```python
from build123d import *

# Parameters (mm, degrees)
SKETCH_1_W          = 60
SKETCH_1_H          = 10.5
SKETCH_1_R          = 1.55
EXTRUDE_1_DEPTH     = 77
SKETCH_2_W          = 25
SKETCH_2_H          = 77
EXTRUDE_2_DEPTH     = 8.5
FILLET_2_R          = 4
SKETCH_3_R          = 1.55
CUT_EXTRUDE_1_DEPTH = 8
SKETCH_4_R          = 2.05
CUT_EXTRUDE_2_DEPTH = 5
CUT_EXTRUDE_START   = -5
SKETCH_5_R          = 2.05
CUT_EXTRUDE_3_DEPTH = 5
FILLET_3_R          = 1
SKETCH_6_R          = 2.05
CUT_EXTRUDE_4_DEPTH = 5


with BuildPart() as part:
    # 草图1 → 凸台-拉伸1 (new body)
    with BuildSketch(Plane.XY):
        with Locations((30, 5.25)):
            Rectangle(SKETCH_1_W, SKETCH_1_H)
        with Locations((15, 5.5)):
            Circle(SKETCH_1_R, mode=Mode.SUBTRACT)
        with Locations((45, 5.5)):
            Circle(SKETCH_1_R, mode=Mode.SUBTRACT)
    extrude(amount=EXTRUDE_1_DEPTH)

    # 草图2 → 凸台-拉伸2 (add)
    with BuildSketch(Plane.XZ):
        with Locations((47.5, 38.5)):
            Rectangle(SKETCH_2_W, SKETCH_2_H)
    extrude(amount=EXTRUDE_2_DEPTH)

    # 圆角2
    fillet_2_edges = [part.edges().sort_by_distance(p)[0] for p in [
        (35, 0, 38.5),
        (60, -8.5, 38.5),
        (35, -8.5, 38.5),
        (0, 10.5, 38.5),
        (60, 10.5, 38.5),
        (0, 0, 38.5),
    ]]
    fillet(fillet_2_edges, radius=FILLET_2_R)

    # 草图3 → 切除-拉伸1 (cut)
    with BuildSketch(Plane.XZ):
        with Locations((11.15, 63.5)):
            Circle(SKETCH_3_R)
        with Locations((11.15, 13.5)):
            Circle(SKETCH_3_R)
        with Locations((25.15, 63.5)):
            Circle(SKETCH_3_R)
        with Locations((25.15, 13.5)):
            Circle(SKETCH_3_R)
    extrude(amount=-CUT_EXTRUDE_1_DEPTH, mode=Mode.SUBTRACT)

    # 草图4 → 切除-拉伸2 (cut)
    with BuildSketch(Plane(origin=(0, 0, 0), x_dir=(-1, 0, 0), z_dir=(0, 0, -1))):
        with Locations((-45, 5.5)):
            Circle(SKETCH_4_R)
        with Locations((-15, 5.5)):
            Circle(SKETCH_4_R)
    extrude(amount=-CUT_EXTRUDE_2_DEPTH, mode=Mode.SUBTRACT)

    # 草图5 → 切除-拉伸3 (cut)
    with BuildSketch(Plane.XY.offset(77).offset(CUT_EXTRUDE_START)):
        with Locations(Location((15, 5.5, 0), (0, 0, 180))):
            Circle(SKETCH_5_R)
        with Locations(Location((45, 5.5, 0), (0, 0, 180))):
            Circle(SKETCH_5_R)
    extrude(amount=CUT_EXTRUDE_3_DEPTH, mode=Mode.SUBTRACT)

    # 圆角3
    fillet_3_edges = [part.edges().sort_by_distance(p)[0] for p in [
        (47.5, -8.5, 77),
        (47.5, -8.5, 0),
        (0, 5.25, 0),
        (30, 10.5, 0),
        (60, 1, 0),
        (35, -4.25, 0),
        (17.5, 0, 0),
        (1.171572875, 9.328427125, 0),
        (1.171572875, 1.171572875, 0),
        (58.828427125, 9.328427125, 0),
        (58.828427125, -7.328427125, 0),
        (36.171572875, -7.328427125, 0),
        (35, -4.25, 77),
        (0, 5.25, 77),
        (17.5, 0, 77),
        (60, 1, 77),
        (30, 10.5, 77),
        (1.171572875, 9.328427125, 77),
        (1.171572875, 1.171572875, 77),
        (58.828427125, 9.328427125, 77),
        (58.828427125, -7.328427125, 77),
        (36.171572875, -7.328427125, 77),
        (33.828427125, -1.171572875, 0),
        (33.828427125, -1.171572875, 77),
    ]]
    fillet(fillet_3_edges, radius=FILLET_3_R)

    # 草图6 → 切除-拉伸4 (cut)
    with BuildSketch(Plane.XZ):
        with Locations((11.15, 63.5)):
            Circle(SKETCH_6_R)
        with Locations((25.15, 63.5)):
            Circle(SKETCH_6_R)
        with Locations((25.15, 13.5)):
            Circle(SKETCH_6_R)
        with Locations((11.15, 13.5)):
            Circle(SKETCH_6_R)
    extrude(amount=-CUT_EXTRUDE_4_DEPTH, mode=Mode.SUBTRACT)


solid = part.part
```
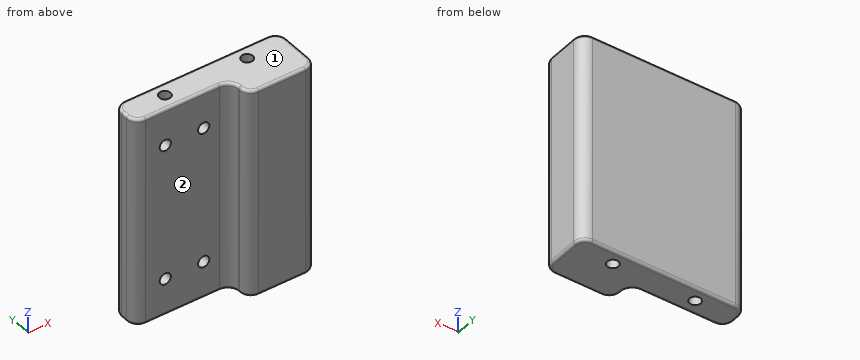
For this review, take the finished solid that the model builds, in its own axes (mm). Face numbers are marked on the shaded views. A direction names the side the tool comes from. Coordinates: 2 decimals unless noted, no trailing zeros. Loops run counter-clockwise (first coordinate to the right, second up) from the corner with the lowest first, then second, coordinate; pieces in that order, holes last. Notation, with made-up numbers: (18.25, -34.75) -> (76.25, -34.75) arc R14 ccw to (76.25, -14.75) -> close; hole circle Ø7 at (11, 39). An arc over 180 degrees is marked (long way). Return JSON: item names as keys, results as strings. Group by question number.
(1) Consider section B-B, the plane z = 13.5. Count the separate pieces of the cut face and the enclosed holes in it, plus the area to 3 significant figures.
(2) Consider section C-C, the plane x = 11.15. Give the boundary of the cut face in (y, z).
(3) Tool access review of the marked faces 1 and 2: name each direction out of +Z, -Z, +X, -X, +Y, -Y from which nothing blocks a thin tool from reaching the whole face with its end or side.
(4) Consider section D-D, the plane z = 46. Give the boundary of the cut face in (x, y).
(5) Consider section A-A, the plane x = 45. Give the boundary of the cut face in (y, z), plus the area to 3 significant figures.
(6) To check wall thickness, follow L1, parallel to Z at x = 25.15, y = 2.6; L2, parallel to X at y = 5.75, z = 56.5; L3, parallel to X at y = 5.5, z = 74.75. State the ranges of each line that lie inside material, in increasing order.
(7) For pin 1 Ø1.5 at (x, z) = (19, 50) entering from -Y; pin 2 Ø1.2 at (x, y) = (44, 5) entering from -Z; pin 3 Ø2 at (x, z) = (10.5, 63.5) entering from -Y, all flat-tipped, find the tip position at first contact; note any pin that passes through.
Results below:
{
 "1": {"separate pieces": "1", "enclosed holes": "2", "area": "754 mm2"},
 "2": {"outline": "(0, 1) arc R1 ccw to (1, 0) -> (9.5, 0) arc R1 ccw to (10.5, 1) -> (10.5, 76) arc R1 ccw to (9.5, 77) -> (1, 77) arc R1 ccw to (0, 76) -> (0, 65.55) -> (5, 65.55) -> (5, 65.05) -> (8, 65.05) -> (8, 61.95) -> (5, 61.95) -> (5, 61.45) -> (0, 61.45) -> (0, 15.55) -> (5, 15.55) -> (5, 15.05) -> (8, 15.05) -> (8, 11.95) -> (5, 11.95) -> (5, 11.45) -> (0, 11.45) -> close"},
 "3": {"face 1": "+Z, +X, -X, +Y, -Y", "face 2": "+Z, -Z, -X, -Y"},
 "4": {"outline": "(0, 4) arc R4 ccw to (4, 0) -> (31, 0) arc R4 cw to (35, -4) -> (35, -4.5) arc R4 ccw to (39, -8.5) -> (56, -8.5) arc R4 ccw to (60, -4.5) -> (60, 6.5) arc R4 ccw to (56, 10.5) -> (4, 10.5) arc R4 ccw to (0, 6.5) -> close; hole circle Ø3.1 at (15, 5.5); hole circle Ø3.1 at (45, 5.5)"},
 "5": {"outline": "(-8.5, 1) arc R1 ccw to (-7.5, 0) -> (3.45, 0) -> (3.45, 5) -> (3.95, 5) -> (3.95, 72) -> (3.45, 72) -> (3.45, 77) -> (-7.5, 77) arc R1 ccw to (-8.5, 76) -> close; (7.05, 5) -> (7.55, 5) -> (7.55, 0) -> (9.5, 0) arc R1 ccw to (10.5, 1) -> (10.5, 76) arc R1 ccw to (9.5, 77) -> (7.55, 77) -> (7.55, 72) -> (7.05, 72) -> close", "area": "1,210 mm2"},
 "6": {"L1": "z = 0 to 11.45, 15.55 to 61.45, 65.55 to 77", "L2": "x = 0 to 13.47, 16.53 to 43.47, 46.53 to 60", "L3": "x = 0 to 12.95, 17.05 to 42.95, 47.05 to 60"},
 "7": {"pin 1": "stops at y = 0", "pin 2": "stops at z = 5", "pin 3": "stops at y = 5"}
}
